Could you check a few things on this model? Use its own coordinates, in mm. Face numbers are marked on the shaded views. A direction names the side the tool comes from. Give positions to 0.01 mm unless a question says otherwise; leave off trailing zeros. Write each loop counter-clockwise with the first axis right and the second up, starting at its lowest first coordinate (ties: lowest second). Pieces come first, ordered by that corner, then holes. Notation, with made-up numbers: M 11.5,15 L 60.5,15 A19 ccw 60.5,22 Z; hole C -28,64.25 d10. An arc over 180 degrees is marked long. One line per item, written item: value.
```python
from build123d import *
from build123d.topology import SkipClean

# Parameters (mm, degrees)
SKETCH2_R                            = 8
SKETCH2_R_2                          = 5
BOSS_EXTRUDE1_DEPTH                  = 8
BOSS_EXTRUDE2_REACH                  = 15.856
BOSS_EXTRUDE2_END_RADIUS             = 8
SKETCH3_R                            = 2.25
BOSS_EXTRUDE2_DIRECTION_2_REACH      = 15.856
BOSS_EXTRUDE2_DIRECTION_2_END_RADIUS = 8
SKETCH4_R                            = 5
CUT_EXTRUDE1_DEPTH                   = 23.978250708
CUT_EXTRUDE2_DEPTH                   = 23.978250708
CUT_EXTRUDE2_DEPTH_BACK              = 23.978250708
SKETCH5_W                            = 10
SKETCH5_H                            = 12
CUT_EXTRUDE3_DEPTH                   = 23.978250708
CUT_EXTRUDE3_DEPTH_BACK              = 23.978250708
SKETCH6_R                            = 1.5
CUT_EXTRUDE4_DEPTH                   = 23.978250752
CUT_EXTRUDE4_DEPTH_BACK              = 23.978250752


with BuildPart() as part:
    # Sketch2 → Boss-Extrude1 (new body)
    with BuildSketch(Plane(origin=(0, 0, 0), x_dir=(1, 0, 0), z_dir=(0, 1, 0))):
        with Locations(Location((0, 0, 0), (0, 0, 270))):
            Circle(SKETCH2_R)
        with Locations(Location((0, 0, 0), (0, 0, 270))):
            Circle(SKETCH2_R_2, mode=Mode.SUBTRACT)
    extrude(amount=BOSS_EXTRUDE1_DEPTH)

    # Boss-Extrude2: up to this cylinder (the profile starts inside it)
    boss_extrude2_end = Plane(origin=(0, 11.750122, 0), z_dir=(0, -1, 0)) * Cylinder(BOSS_EXTRUDE2_END_RADIUS, 48.712, mode=Mode.PRIVATE)
    # Sketch3 → Boss-Extrude2 (add, up to the surface)
    with BuildSketch(Plane.XY, mode=Mode.PRIVATE) as boss_extrude2_sk1:
        with BuildLine():
            Line((0, 8), (-4.5, 8))
            add(Edge.make_bspline(
                [(-4.5, 15.5), (0, 11.75), (-4.5, 8)],
                knots=[0, 0, 0, 1, 1, 1], degree=2))
            ThreePointArc((-4.5, 15.5), (0, 20), (4.5, 15.5))
            add(Edge.make_bspline(
                [(4.5, 15.5), (0, 11.75), (4.5, 8)],
                knots=[0, 0, 0, 1, 1, 1], degree=2))
            Line((4.5, 8), (0, 8))
        make_face()
        with Locations(Location((0, 15.5, 0), (0, 0, 180))):
            Circle(SKETCH3_R, mode=Mode.SUBTRACT)
    boss_extrude2_tool1 = extrude(boss_extrude2_sk1.sketch, amount=BOSS_EXTRUDE2_REACH, mode=Mode.PRIVATE) & boss_extrude2_end
    add(boss_extrude2_tool1.solids().sort_by_distance((2.1, 11.750122, 0))[0])

    # Boss-Extrude2 direction 2: up to this cylinder (the profile starts inside it)
    boss_extrude2_direction_2_end = Plane(origin=(0, 11.750122, 0), z_dir=(0, -1, 0)) * Cylinder(BOSS_EXTRUDE2_DIRECTION_2_END_RADIUS, 48.712, mode=Mode.PRIVATE)
    # Sketch3 → Boss-Extrude2 direction 2 (add, up to the surface)
    with BuildSketch(Plane.XY, mode=Mode.PRIVATE) as boss_extrude2_direction_2_sk1:
        with BuildLine():
            Line((0, 8), (-4.5, 8))
            add(Edge.make_bspline(
                [(-4.5, 15.5), (0, 11.75), (-4.5, 8)],
                knots=[0, 0, 0, 1, 1, 1], degree=2))
            ThreePointArc((-4.5, 15.5), (0, 20), (4.5, 15.5))
            add(Edge.make_bspline(
                [(4.5, 15.5), (0, 11.75), (4.5, 8)],
                knots=[0, 0, 0, 1, 1, 1], degree=2))
            Line((4.5, 8), (0, 8))
        make_face()
        with Locations(Location((0, 15.5, 0), (0, 0, 180))):
            Circle(SKETCH3_R, mode=Mode.SUBTRACT)
    boss_extrude2_direction_2_tool1 = extrude(boss_extrude2_direction_2_sk1.sketch, amount=-BOSS_EXTRUDE2_DIRECTION_2_REACH, mode=Mode.PRIVATE) & boss_extrude2_direction_2_end
    add(boss_extrude2_direction_2_tool1.solids().sort_by_distance((2.1, 11.750122, 0))[0])

    # Sketch4 → Cut-Extrude1 (cut, through all)
    with BuildSketch(Plane.XZ):
        with Locations(Location((0, 0, 0), (0, 0, 90))):
            Circle(SKETCH4_R)
    extrude(amount=-CUT_EXTRUDE1_DEPTH, mode=Mode.SUBTRACT)

    # Sketch5 → Cut-Extrude2 (cut, two sides: drawn at the far end of the back side and taken through both)
    with BuildSketch(Plane(origin=(0, 0, 0), x_dir=(0, 0, -1), z_dir=(1, 0, 0)).offset(-CUT_EXTRUDE2_DEPTH_BACK)):
        with Locations((0, 14)):
            Rectangle(SKETCH5_W, SKETCH5_H)
    extrude(amount=CUT_EXTRUDE2_DEPTH + CUT_EXTRUDE2_DEPTH_BACK, mode=Mode.SUBTRACT)

    # Sketch6 → Cut-Extrude3 (cut, two sides: drawn at the far end of the back side and taken through both)
    with SkipClean():  # the faces are left unmerged after this step: merging them gives an invalid solid
        with BuildSketch(Plane.XY.offset(-CUT_EXTRUDE3_DEPTH_BACK)):
            with Locations((0, 4)):
                Circle(SKETCH6_R)
        extrude(amount=CUT_EXTRUDE3_DEPTH + CUT_EXTRUDE3_DEPTH_BACK, mode=Mode.SUBTRACT)

    # Sketch7 → Cut-Extrude4 (cut, two sides: drawn at the far end of the back side and taken through both)
    with SkipClean():  # the faces are left unmerged after this step: merging them gives an invalid solid
        with BuildSketch(Plane.XY.offset(-CUT_EXTRUDE4_DEPTH_BACK)):
            with BuildLine():
                Line((-3.112474899, 18.75), (3.112474899, 18.75))
                ThreePointArc((3.112474899, 18.75), (0, 20), (-3.112474899, 18.75))
            make_face()
        extrude(amount=CUT_EXTRUDE4_DEPTH + CUT_EXTRUDE4_DEPTH_BACK, mode=Mode.SUBTRACT)


solid = part.part
```
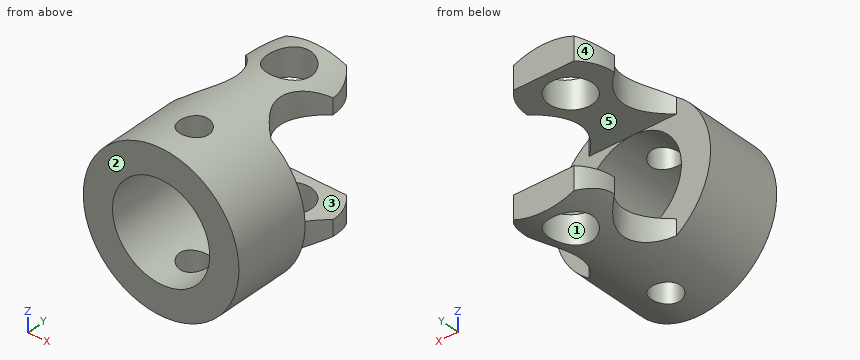
1) If we section it at B-B, the plane x = -1.75: Write out the boundary of the cut face in (y, z), then the cut area to 3 significant figures.
Outcome:
outline: M 0,-7.81 L 14.09,-7.81 L 14.09,-5 L 8,-5 L 8,-4.68 L 0,-4.68 Z; M 0,4.68 L 8,4.68 L 8,5 L 14.09,5 L 14.09,7.81 L 0,7.81 Z; M 16.91,-7.81 L 18.75,-7.81 L 18.75,-5 L 16.91,-5 Z; M 16.91,5 L 18.75,5 L 18.75,7.81 L 16.91,7.81 Z
area: 94.4 mm^2
2) If we section it at D-D, the plane y = 2: Write out the boundary of the cut face in (x, z).
Outcome:
outline: C 0,0 d16; hole C 0,0 d10
3) I'm going to push flat-ended pins straight in: pin 1 (6 mm diameter, centred on y = 16.5, z = -3, fed in from +X); pin 2 (2.5 mm diameter, centred on x = 4, z = -0.5, fed in from +Y); pin 3 (8 mm diameter, centred on y = 5, z = 5, fed in from -X). Where does each tip first touch, or does it pass through?
Outcome:
pin 1: stops at x = 4.5
pin 2: stops at y = 8
pin 3: stops at x = -7.94
4) We'd pull the mould along Y, two halves only. Please class the marked faces 1, 2 and 3: pulls with the +Y half, pulls with the -Y half, needs draft (parallel to the pull), parting line crosses it, or undercut.
Outcome:
face 1: undercut
face 2: pulls with the -Y half
face 3: needs draft
5) If we section it at C-C, the plane y = 4: Write out the boundary of the cut face in (x, z).
Outcome:
outline: M -1.5,-7.86 L -1.5,-4.77 A5 cw -1.5,4.77 L -1.5,7.86 A8 ccw Z; M 1.5,-7.86 A8 ccw 1.5,7.86 L 1.5,4.77 A5 cw 1.5,-4.77 Z
6) Please list where these lines run through material, in increasing order: L1, parallel to Y at x = 0, z = 6.7; L2, parallel to Z at x = 0.25, y = 13; L3, parallel to Z at x = 3.75, y = 15. Write a range as from..to.
Outcome:
L1: y = 0..2.5, 5.5..13.25, 17.75..18.75
L2: z = -8..-5, 5..8
L3: z = -7.07..-5, 5..7.07
7) If we section it at A-A, the plane z = 0: Write out the boundary of the cut face in (x, y).
Outcome:
outline: M -8,0 L -5,0 L -5,8 L -8,8 Z; M 5,0 L 8,0 L 8,8 L 5,8 Z
8) On a 3-axis mill with a long thin cutter (end or side, diameter ignored), from which of +Z, -Z, +X, -X, +Y, -Y can I reach the whole of each face in a straight line? I mean the marked faces 4 and 5. Say none if no direction works.
Outcome:
face 4: +Z, -Z, -X, +Y
face 5: +X, -X, +Y
